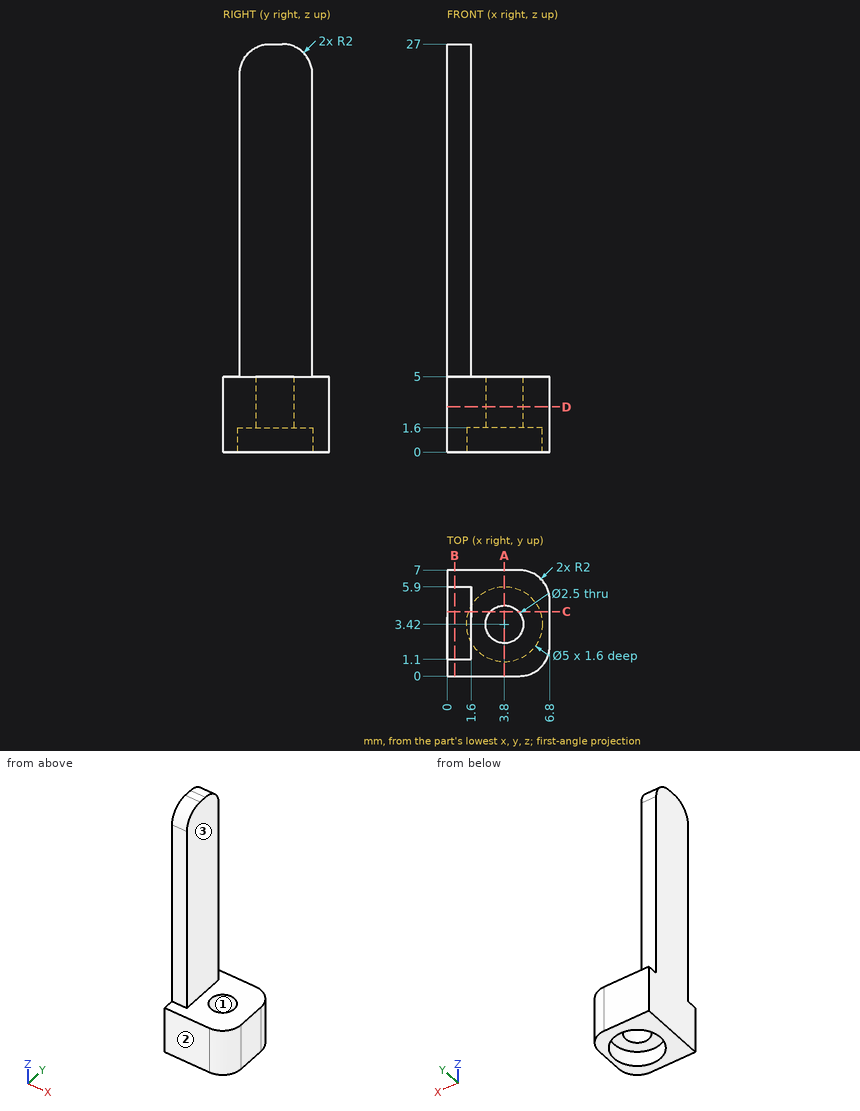
Part print with two shaded views. Sizes in mm from the minimum x, y, z corner. Round coordinates to 2 decimals unless told otherwise and drop trailing zeros. Order: outer loops, then holes, each group sorted by start corner. A loop starts at its lowest first (then second) coordinate and runs counter-clockwise, first axis right, second up.
(1) Band-saw the part on A-A (x = 3.8). List the corners of the cut face in (y, z).
(2) Drill centre lines: line 1 (Y direction, x = 3.8, z = 2.6); line 2 (Y direction, x = 3.8, z = 0.7); line 3 (Z direction, x = 3.5, y = 0.75). Where is each one in solid material? Low to high.
(3) Band-saw the part on D-D (z = 3). List the corners of the cut face in (x, y).
(4) Band-saw the part on B-B (x = 0.5). List the corners of the cut face in (y, z).
(5) Pull direction X, two halves, no side cores. Call the marked faces 1, 2 and 3: released by +X, released by -X, zero draft, split by the parting line, or undercut.
(6) Pin check, flat tips, straight feed: pin 1 (0.5 mm diameter, centred on x = 1, z = 12, fed in from -Y); pin 2 (0.8 mm diameter, centred on x = 0.5, z = 11, fed in from +Y); pin 3 (3 mm diameter, centred on x = 1, y = 1.5, fed in from +Z). Stop position of each tip, or through.
(7) Band-saw the part on C-C (y = 4.25). List the corners of the cut face in (x, z).
Verdict:
1. outline: (0, 0) - (0.92, 0) - (0.92, 1.6) - (2.17, 1.6) - (2.17, 5) - (0, 5) - close; (4.67, 1.6) - (5.92, 1.6) - (5.92, 0) - (7, 0) - (7, 5) - (4.67, 5) - close
2. line 1: y = 0 to 2.17, 4.67 to 7
2. line 2: y = 0 to 0.92, 5.92 to 7
2. line 3: z = 0 to 5
3. outline: (0, 0) - (4.8, 0) arc R2 ccw to (6.8, 2) - (6.8, 5) arc R2 ccw to (4.8, 7) - (0, 7) - close; hole circle Ø2.5 at (3.8, 3.42)
4. outline: (0, 0) - (7, 0) - (7, 5) - (5.9, 5) - (5.9, 25) arc R2 ccw to (3.9, 27) - (3.1, 27) arc R2 ccw to (1.1, 25) - (1.1, 5) - (0, 5) - close
5. face 1: undercut
5. face 2: zero draft
5. face 3: released by +X
6. pin 1: stops at y = 1.1
6. pin 2: stops at y = 5.9
6. pin 3: stops at z = 27
7. outline: (0, 0) - (1.44, 0) - (1.44, 1.6) - (2.87, 1.6) - (2.87, 5) - (1.6, 5) - (1.6, 26.97) - (0, 26.97) - close; (4.73, 1.6) - (6.16, 1.6) - (6.16, 0) - (6.8, 0) - (6.8, 5) - (4.73, 5) - close
